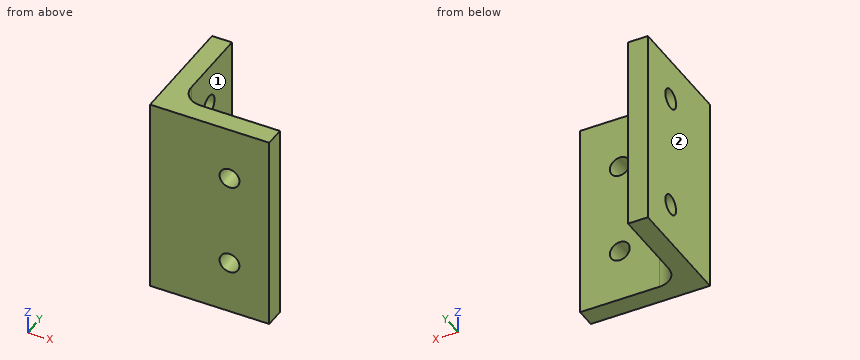
Autodesk Fusion 360 part; units mm, degrees
sketch "Boceto1" plane through (0, 0, 0) normal (0, 0, 1) x (1, 0, 0)
  line L0 (0, 0) -> (3, 0)
  line L1 (3, 0) -> (3, 22.4)
  line L2 (3, 22.4) -> (0, 22.4)
  line L3 (0, 22.4) -> (0, 0)
  dimension "d1" = 3
  dimension "d2" = 22.4
extrude "Extruir1" add sketch "Boceto1" along normal blind 30
sketch "Boceto2" plane through (3, 0, 0) normal (1, 0, 0) x (0, 0, -1)
  line L0 (0, 0) -> (0, 22.4)
  line L1 (0, 22.4) -> (-30, 22.4)
  line L2 (-30, 22.4) -> (-30, 0)
  line L3 (-30, 0) -> (0, 0)
  circle A0 centre (-23.75, 11) radius 1.65
  circle A1 centre (-6.25, 11) radius 1.65
  dimension "d7" = 3.3
  dimension "d8" = 3.3
hole "Agujero1" at (3, 11, 23.75) at (3, 11, 6.25) direction (-1, 0, 0) diameter 3 depth 10 tip angle 118
sketch "Boceto3" plane through (3, 0, 0) normal (1, 0, 0) x (0, 0, -1)
  circle A0 centre (-23.75, 11) radius 1.5
  circle A1 centre (-6.25, 11) radius 1.5
  line L0 (0, 0) -> (0, 22.4)
  line L1 (0, 22.4) -> (-30, 22.4)
  line L2 (-30, 22.4) -> (-30, 0)
  line L3 (-30, 0) -> (0, 0)
  line L4 (-30, 0) -> (0, 0)
  line L5 (0, 0) -> (0, 3)
  line L6 (0, 3) -> (-30, 3)
  line L7 (-30, 3) -> (-30, 0)
  dimension "d12" = 30
  dimension "d13" = 3
extrude "Extruir2" add sketch "Boceto3" along normal blind 15 contours L0 L2 L3 L4 L5 L6 L7
fillet "Empalme1" radius 3 1 edges at (3, 3, 15)
sketch "Boceto4" plane through (0, 3, 0) normal (0, 1, 0) x (-1, 0, 0)
  line L0 (-6, 0) -> (-6, 30)
  line L1 (-6, 30) -> (-18, 30)
  line L2 (-18, 30) -> (-18, 0)
  line L3 (-18, 0) -> (-6, 0)
  circle A0 centre (-12, 8) radius 1.5
  circle A1 centre (-12, 22) radius 1.5
  dimension "d18" = 3
  dimension "d19" = 3
hole "Agujero2" at (12, 3, 22) at (12, 3, 8) direction (0, -1, 0) diameter 3 depth 10 tip angle 118
sketch "Boceto5" plane through (3, 0, 0) normal (1, 0, 0) x (0, 0, -1)
  line L0 (-30, 6) -> (0, 6)
  line L1 (0, 6) -> (0, 22.4)
  line L2 (0, 22.4) -> (-30, 22.4)
  line L3 (-30, 22.4) -> (-30, 6)
  circle A0 centre (-23.75, 11) radius 1.5
  circle A1 centre (-6.25, 11) radius 1.5
  line L4 (-30, 22.4) -> (0, 22.4)
  line L5 (0, 22.4) -> (0, 17.4)
  line L6 (0, 17.4) -> (-30, 17.4)
  line L7 (-30, 17.4) -> (-30, 22.4)
  dimension "d23" = 5
extrude "Extruir3" cut sketch "Boceto5" against normal blind 9 contours L1 L2 L3 L4 L5 L6 L7
Model file for the job. Use its own axes, mm. Face numbers are marked on the shaded views. A direction names the side the tool comes from. Round coordinates to 2 decimals unless told otherwise and drop trailing zeros. Loops run counter-clockwise (first coordinate to the right, second up) from the corner with the lowest first, then second, coordinate; pieces in that order, holes last. Notation, with made-up numbers: M 84.25,88.5 L 121.25,88.5 A19 ccw 121.25,115.5 Z; hole C 84.25,-7.5 d4. An arc over 180 degrees is marked long. Put each result on its own line as item: value. Start each with the question number.
Item 1: Cut at D-D (y = 14.75). List the corners of the cut face in (x, z).
Item 2: Cut at B-B (x = 12). List the corners of the cut face in (y, z), then the cut area to 3 significant figures.
Item 3: Cut at A-A (y = 11). List the corners of the cut face in (x, z), then the cut area to 3 significant figures.
Item 4: Drill centre lines: line 1 along Z through (x, y) = (0.8, 11); line 2 along Z through (x, y) = (12, 1.05); line 3 along Y through (x, z) = (2.3, 23.75). Where is each one in solid material? Low to high.
Item 5: 3-axis set-ups, long thin cutter, end or side, ignore diameter. For the marked faces 1 and 2: which of +Z, -Z, +X, -X, +Y, -Y reach the whole face in a straight line?
Item 6: Drop flat-ended pins along their axis: P1, Ø4, axis at y = 11, z = 23.75, coming from the +X side; P2, Ø9.5, axis at x = 14, z = 10, coming from the +Y side; P3, Ø6, axis at y = 8, z = 4.5, coming from the +X side. Give the stop position or say it passes through.
Item 7: Cut at C-C (z = 14.5). List the corners of the cut face in (x, y), then the cut area to 3 significant figures.
Answer block:
1. outline: M 0,0 L 3,0 L 3,30 L 0,30 Z
2. outline: M 0,0 L 3,0 L 3,6.5 L 0,6.5 Z; M 0,9.5 L 3,9.5 L 3,20.5 L 0,20.5 Z; M 0,23.5 L 3,23.5 L 3,30 L 0,30 Z
2. area: 72.0 mm2
3. outline: M 0,0 L 3,0 L 3,4.75 L 0,4.75 Z; M 0,7.75 L 3,7.75 L 3,22.25 L 0,22.25 Z; M 0,25.25 L 3,25.25 L 3,30 L 0,30 Z
3. area: 72.0 mm2
4. line 1: 0 to 4.75, 7.75 to 22.25, 25.25 to 30
4. line 2: 0 to 6.5, 9.5 to 20.5, 23.5 to 30
4. line 3: 0 to 9.5, 12.5 to 17.4
5. face 1: +Z, -Z, +X, +Y
5. face 2: +Z, -Z, -X, +Y, -Y
6. P1: x = 3
6. P2: y = 3
6. P3: x = 3.17
7. outline: M 0,0 L 18,0 L 18,3 L 6,3 A3 cw 3,6 L 3,17.4 L 0,17.4 Z
7. area: 99.1 mm2
